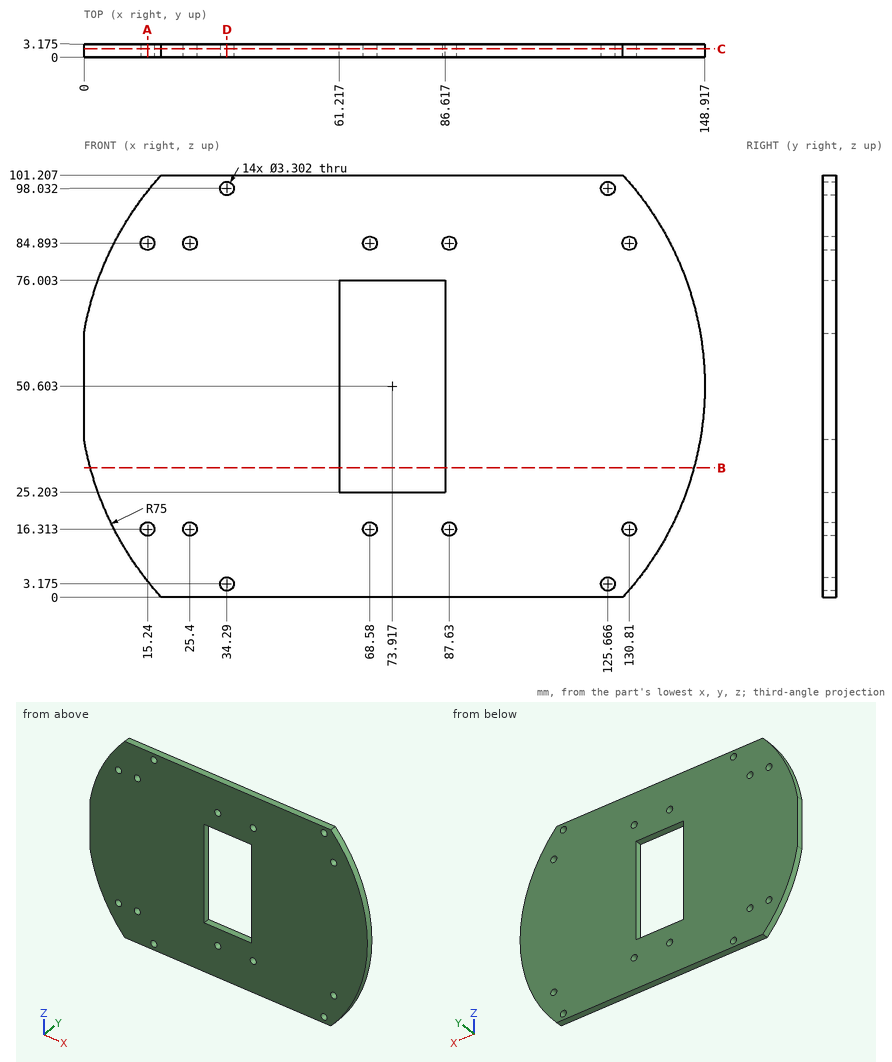
Source: three-view drawing plus pictorial views. Frame: mm from the lowest corner of the part. Give positions to 0.01 mm unless a question says otherwise; leave off trailing zeros. Order: outer loops, then holes, each group sorted by start corner. A loop starts at its lowest first (then second) coordinate and runs counter-clockwise, first axis right, second up. Notation, with made-up numbers: (15.25, 53) - (74.25, 53) arc R21 cw to (74.25, 89) - close; hole circle Ø10 at (39, -24). An arc over 180 degrees is marked (long way). Answer as a JSON object with one key per item and string values. Group by question number.
Q1. First-contact query: pin 1 Ø1 at (y, z) = (2, 52) entering from +X. Flat tip, straight axial feed; report the tip coordinate or a pass-through.
Q2. Cut plane B-B, the plane z = 31. Output: boundary loops of the cut face in (x, y) (1 decimal), then the cut area to 3 significant figures.
Q3. Cut plane C-C, the plane y = 2. Count the separate pieces of the cut face and the enclosed holes in it, then the cut area to 3 significant figures.
Q4. Cut plane A-A, the plane x = 15.24. Output: boundary loops of the cut face in (y, z) (1 decimal).
Q5. Line query: probe 1 along Z at (x, y) = (79, 2.7); probe 2 along Z at (x, y) = (89, 2.6) (1 decimal); probe 3 along X at (y, z) = (1.2, 85.5) (1 decimal). Output: solid intervals per line, ascending.
Q6. Cut plane D-D, the plane x = 34.29. Output: boundary loops of the cut face in (y, z) (1 decimal).
Results:
{
 "1": {"pin 1": "x = 148.91"},
 "2": {"outline": "(1.5, 0) - (61.2, 0) - (61.2, 3.2) - (1.5, 3.2) - close; (86.6, 0) - (146.3, 0) - (146.3, 3.2) - (86.6, 3.2) - close", "area": "379 mm^2"},
 "3": {"separate pieces": "1", "enclosed holes": "15", "area": "12,500 mm^2"},
 "4": {"outline": "(0, 3.9) - (3.2, 3.9) - (3.2, 14.7) - (0, 14.7) - close; (0, 18) - (3.2, 18) - (3.2, 83.2) - (0, 83.2) - close; (0, 86.5) - (3.2, 86.5) - (3.2, 97.3) - (0, 97.3) - close"},
 "5": {"probe 1": "0 to 25.2, 76 to 101.21", "probe 2": "0 to 15.4, 17.2 to 84, 85.8 to 101.2", "probe 3": "7.5 to 13.7, 16.8 to 23.9, 26.9 to 67, 70.1 to 86.1, 89.2 to 129.3, 132.3 to 140.3"},
 "6": {"outline": "(0, 0) - (3.2, 0) - (3.2, 1.5) - (0, 1.5) - close; (0, 4.8) - (3.2, 4.8) - (3.2, 96.4) - (0, 96.4) - close; (0, 99.7) - (3.2, 99.7) - (3.2, 101.2) - (0, 101.2) - close"}
}
